Verification items for the finished model (mm, model axes). Give positions to 0.01 mm unless a question says otherwise; leave off trailing zeros. Write each loop counter-clockwise with the first axis right and the second up, starting at its lowest first coordinate (ties: lowest second). Pieces come first, ordered by that corner, then holes.
Autodesk Inventor part; units mm, degrees
ref_plane "YZ Plane" through (0, 0, 0) normal (1, 0, 0) x (0, 1, 0)
ref_plane "XZ Plane" through (0, 0, 0) normal (0, 1, 0) x (-1, 0, 0)
ref_plane "XY Plane" through (0, 0, 0) normal (0, 0, 1) x (1, 0, 0)
sketch "스케치3" plane through (0, 0, 0) normal (0, 1, 0) x (-1, 0, 0)
  line L0 (68.3838, -28.3255) -> (28.3255, -68.3838)
  line L1 (28.3255, -68.3838) -> (-28.3255, -68.3838)
  line L2 (-28.3255, -68.3838) -> (-68.3838, -28.3255)
  line L3 (-68.3838, -28.3255) -> (-68.3838, 28.3255)
  line L4 (-68.3838, 28.3255) -> (-28.3255, 68.3838)
  line L5 (-28.3255, 68.3838) -> (28.3255, 68.3838)
  line L6 (28.3255, 68.3838) -> (68.3838, 28.3255)
  line L7 (68.3838, 28.3255) -> (68.3838, -28.3255)
  line L8 (65.1838, -27) -> (27, -65.1838)
  line L9 (27, -65.1838) -> (-27, -65.1838)
  line L10 (-27, -65.1838) -> (-65.1838, -27)
  line L11 (-65.1838, -27) -> (-65.1838, 27)
  line L12 (-65.1838, 27) -> (-27, 65.1838)
  line L13 (-27, 65.1838) -> (27, 65.1838)
  line L14 (27, 65.1838) -> (65.1838, 27)
  line L15 (65.1838, 27) -> (65.1838, -27)
  point P0 (0, 0)
  point P1 (0, 0)
  point P2 (0, 0)
  point P3 (0, 0)
  dimension "d43" = 54
  dimension "d44" = 3.2
extrude "돌출2" add sketch "스케치3" along normal blind 6.8 contours L0 L1 L2 L3 L4 L5 L6 L7 | L8 L9 L10 L11 L12 L13 L14 L15
sketch "스케치4" plane through (0, 6.8, 0) normal (0, 1, 0) x (1, 0, 0)
  line L0 (26.9172, -64.9838) -> (-26.9172, -64.9838)
  line L1 (-26.9172, -64.9838) -> (-64.9838, -26.9172)
  line L2 (-64.9838, -26.9172) -> (-64.9838, 26.9172)
  line L3 (-64.9838, 26.9172) -> (-26.9172, 64.9838)
  line L4 (-26.9172, 64.9838) -> (26.9172, 64.9838)
  line L5 (26.9172, 64.9838) -> (64.9838, 26.9172)
  line L6 (64.9838, 26.9172) -> (64.9838, -26.9172)
  line L7 (64.9838, -26.9172) -> (26.9172, -64.9838)
  line L8 (-27.6627, 66.7838) -> (27.6627, 66.7838)
  line L9 (27.6627, 66.7838) -> (66.7838, 27.6627)
  line L10 (66.7838, 27.6627) -> (66.7838, -27.6627)
  line L11 (66.7838, -27.6627) -> (27.6627, -66.7838)
  line L12 (27.6627, -66.7838) -> (-27.6627, -66.7838)
  line L13 (-27.6627, -66.7838) -> (-66.7838, -27.6627)
  line L14 (-66.7838, -27.6627) -> (-66.7838, 27.6627)
  line L15 (-66.7838, 27.6627) -> (-27.6627, 66.7838)
  line L16 (-26.8343, 64.7838) -> (26.8343, 64.7838)
  line L17 (26.8343, 64.7838) -> (64.7838, 26.8343)
  line L18 (64.7838, 26.8343) -> (64.7838, -26.8343)
  line L19 (64.7838, -26.8343) -> (26.8343, -64.7838)
  line L20 (26.8343, -64.7838) -> (-26.8343, -64.7838)
  line L21 (-26.8343, -64.7838) -> (-64.7838, -26.8343)
  line L22 (-64.7838, -26.8343) -> (-64.7838, 26.8343)
  line L23 (-64.7838, 26.8343) -> (-26.8343, 64.7838)
  line L24 (-68.3838, 28.3255) -> (-68.3838, -28.3255)
  point P0 (0, 0)
  point P1 (0, 0)
  point P2 (0, 0)
  point P3 (0, 0)
  dimension "d42" = 1.8
  dimension "d45" = 0.2
  dimension "d60" = 1.6
extrude "돌출3" cut sketch "스케치4" against normal blind 1.2 contours L0 L1 L2 L3 L4 L5 L6 L7 | L8 L9 L10 L11 L12 L13 L14 L15 | L16 L17 L18 L19 L20 L21 L22 L23
sketch "스케치5" plane through (0, 0, 0) normal (0, -1, 0) x (1, 0, 0)
  line L0 (10, 2.5) -> (20, 2.5)
  line L1 (20, 2.5) -> (20, -2.5)
  line L2 (20, -2.5) -> (10, -2.5)
  line L3 (10, -2.5) -> (10, 2.5)
  line L4 (10, 2.5) -> (20, -2.5) construction
  line L5 (20, 2.5) -> (10, -2.5) construction
  line L6 (-20, 2.5) -> (-10, 2.5)
  line L7 (-10, 2.5) -> (-10, -2.5)
  line L8 (-10, -2.5) -> (-20, -2.5)
  line L9 (-20, -2.5) -> (-20, 2.5)
  line L10 (-20, 2.5) -> (-10, -2.5) construction
  line L11 (-10, 2.5) -> (-20, -2.5) construction
  point P0 (0, 0)
  point P1 (15, 0)
  point P2 (-15, 0)
  dimension "d11" = 10
  dimension "d12" = 5
  dimension "d13" = 10
  dimension "d16" = 30
extrude "돌출4" add sketch "스케치5" along normal blind 10
sketch "스케치6" plane through (-10, 0, -2.5) normal (0, 0, -1) x (-1, 0, 0)
  circle A0 centre (5, -10) radius 5
  circle A1 centre (-25, -10) radius 5
  line L0 (-20, -10) -> (-30, -10)
  line L1 (10, -10) -> (0, -10)
  point P0 (-10, 0)
  dimension "d23" = 10
  dimension "d24" = 10
extrude "돌출5" add sketch "스케치6" against normal blind 5
sketch "스케치7" plane through (-10, 0, -2.5) normal (0, 0, -1) x (-1, 0, 0)
  circle A0 centre (5, -10) radius 1.25
  line L0 (10, 0) -> (10, -10)
  line L1 (0, 0) -> (10, 0)
  line L2 (4.7788, 0) -> (0, 0)
  circle A1 centre (-25, -10) radius 1.25
  point P0 (-10, 0)
  dimension "d27" = 2.5
  dimension "d28" = 5
  dimension "d31" = 30
extrude "돌출6" cut sketch "스케치7" against normal blind 5
sketch "스케치8" plane through (0, 0, 0) normal (0, -1, 0) x (1, 0, 0)
  circle A0 centre (0, -35) radius 1.25
  line L0 (-10, 2.5) -> (-10, -2.5)
  point P0 (0, 0)
  point P1 (-10, 0)
  dimension "d38" = 2.5
  dimension "d39" = 35
sketch "스케치9" plane through (0, 5.6, 0) normal (0, 1, 0) x (1, 0, 0)
  line L0 (-26.8343, 64.7838) -> (26.8343, 64.7838)
  line L1 (26.8343, 64.7838) -> (64.7838, 26.8343)
  line L2 (64.7838, 26.8343) -> (64.7838, -26.8343)
  line L3 (64.7838, -26.8343) -> (26.8343, -64.7838)
  line L4 (26.8343, -64.7838) -> (-26.8343, -64.7838)
  line L5 (-26.8343, -64.7838) -> (-64.7838, -26.8343)
  line L6 (-64.7838, -26.8343) -> (-64.7838, 26.8343)
  line L7 (-64.7838, 26.8343) -> (-26.8343, 64.7838)
  line L8 (-27.6627, 66.7838) -> (27.6627, 66.7838)
  line L9 (-25.5917, 61.7838) -> (25.5917, 61.7838)
  line L10 (25.5917, 61.7838) -> (61.7838, 25.5917)
  line L11 (61.7838, 25.5917) -> (61.7838, -25.5917)
  line L12 (61.7838, -25.5917) -> (25.5917, -61.7838)
  line L13 (25.5917, -61.7838) -> (-25.5917, -61.7838)
  line L14 (-25.5917, -61.7838) -> (-61.7838, -25.5917)
  line L15 (-61.7838, -25.5917) -> (-61.7838, 25.5917)
  line L16 (-61.7838, 25.5917) -> (-25.5917, 61.7838)
  point P0 (0, 0)
  point P1 (0, 0)
  point P2 (0, 0)
  dimension "d46" = 2
  dimension "d47" = 3
extrude "돌출8" add sketch "스케치9" along normal blind 0.6 contours L0 L1 L2 L3 L4 L5 L6 L7 | L9 L10 L11 L12 L13 L14 L15 L16
fillet "모깎기1" radius 1.2 16 edges at (-68.3838, 6.8, 0) (-48.3546, 6.8, 48.3546) (0, 6.8, 68.3838) (48.3546, 6.8, 48.3546) (68.3838, 6.8, 0) (48.3546, 6.8, -48.3546) (0, 6.8, -68.3838) (-48.3546, 6.8, -48.3546) (48.3546, 0, 48.3546) (0, 0, 68.3838) (-48.3546, 0, 48.3546) (-68.3838, 0, 0) (-48.3546, 0, -48.3546) (0, 0, -68.3838) (48.3546, 0, -48.3546) (68.3838, 0, 0)
sketch "스케치10" plane through (0, 0, 0) normal (0, -1, 0) x (1, 0, 0)
  line L0 (-20, 2.5) -> (-10, 2.5)
  line L1 (-10, -2.5) -> (-20, -2.5)
  line L2 (-20, 2.5) -> (-19, 2.5)
  line L3 (-19, 2.5) -> (-19, -2.5)
  line L4 (-19, -2.5) -> (-20, -2.5)
  line L5 (-20, -2.5) -> (-20, 2.5)
  line L6 (20, -2.5) -> (10, -2.5)
  line L7 (10, 2.5) -> (20, 2.5)
  line L8 (20, -2.5) -> (19, -2.5)
  line L9 (19, -2.5) -> (19, 2.5)
  line L10 (19, 2.5) -> (20, 2.5)
  line L11 (20, 2.5) -> (20, -2.5)
  point P0 (0, 0)
  dimension "d54" = 1
  dimension "d55" = 1
extrude "돌출9" cut sketch "스케치10" along normal blind 15
extrude "돌출10" cut sketch "스케치8" against normal up to surface (6.2 mm away)
equation "\"d55\" = d54"
properties part number "OV-PAM_top_2"
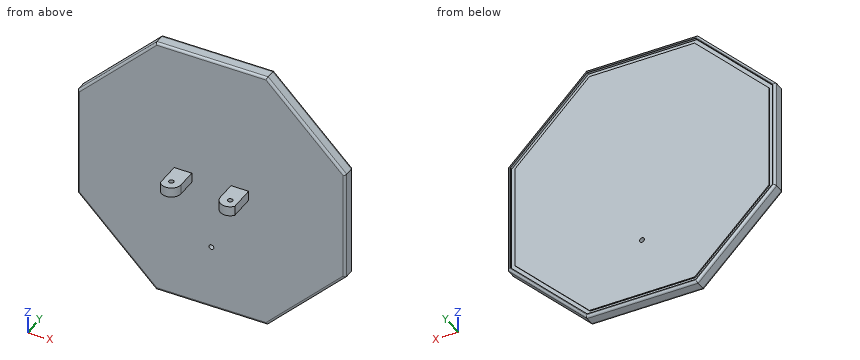
Item 1: Sectioned sample at C-C on x = 21. Record the cut outline in (y, z).
Answer key:
outline: (0, -67.18) arc R1.2 ccw to (1.2, -68.38) - (5.6, -68.38) arc R1.2 ccw to (6.8, -67.18) - (6.8, -66.78) - (5.6, -66.78) - (5.6, -64.78) - (6.2, -64.78) - (6.2, 64.78) - (5.6, 64.78) - (5.6, 66.78) - (6.8, 66.78) - (6.8, 67.18) arc R1.2 ccw to (5.6, 68.38) - (1.2, 68.38) arc R1.2 ccw to (0, 67.18) - close
Item 2: Scan lines: line 1 along Z through (x, y) = (26, 5.75); line 2 along Y through (x, z) = (-15, 0); line 3 along Y through (x, z) = (12.5, 13.5). Record each from-to range of solid material in increasing order.
Answer key:
line 1: z = -68.37 to -66.78, -64.78 to 64.78, 66.78 to 68.37
line 2: y = -15 to -11.25, -8.75 to 6.2
line 3: y = 0 to 6.2
Item 3: Sectioned sample at A-A on y = -4.5. Record the cut outline in (x, z), then the cut area to 3 significant figures.
Answer key:
outline: (-19, -2.5) - (-10, -2.5) - (-10, 2.5) - (-19, 2.5) - close; (10, -2.5) - (19, -2.5) - (19, 2.5) - (10, 2.5) - close
area: 90.0 mm2
Item 4: Sectioned sample at B-B on z = -17.5. Record the cut outline in (x, y).
Answer key:
outline: (-68.38, 1.2) arc R1.2 ccw to (-67.18, 0) - (67.18, 0) arc R1.2 ccw to (68.38, 1.2) - (68.38, 5.6) arc R1.2 ccw to (67.18, 6.8) - (66.78, 6.8) - (66.78, 5.6) - (64.78, 5.6) - (64.78, 6.2) - (-64.78, 6.2) - (-64.78, 5.6) - (-66.78, 5.6) - (-66.78, 6.8) - (-67.18, 6.8) arc R1.2 ccw to (-68.38, 5.6) - close
Item 5: Depth check by flat-ended pin: pin 1 (1 mm diameter, centred on x = 53, z = -39.5, fed in from -Y); pin 2 (1 mm diameter, centred on y = 6.5, z = -13, fed in from +X); pin 3 (0.6 mm diameter, centred on x = 10.5, y = 6.5, fed in from -Z). Enter the tip coordinate at first touch or a pass-through.
Answer key:
pin 1: stops at y = 0
pin 2: stops at x = 68.32
pin 3: stops at z = -68.22
